The model under review builds one solid part; all positions refer to its coordinate system, in mm. A direction names the side the tool comes from. Give positions to 0.01 mm unless a question says otherwise; leave off trailing zeros. Loops run counter-clockwise (first coordinate to the right, second up) from the corner with the lowest first, then second, coordinate; pieces in that order, holes last. Notation, with made-up numbers: M 67,20.5 L 76,20.5 A31 cw 76,56.5 Z; hole C -13,-10 d8. An arc over 180 degrees is marked long. Return JSON: item names as keys, results as strings. Group by question number.
```python
from build123d import *

# Parameters (mm, degrees)
BOSS_EXTRUDE1_DEPTH                       = 10.668
CSK_FOR_6_FLAT_HEAD_MACHINE_SCREW_2_COUNT = 2
CSK_FOR_6_FLAT_HEAD_MACHINE_SCREW_2_PITCH = 29.9974
SKETCH4_R                                 = 1.238307914
CUT_EXTRUDE1_DEPTH                        = 2540


with BuildPart() as part:
    # Sketch1 → Boss-Extrude1 (new body)
    with BuildSketch(Plane.XY.offset(21.5138)):
        with BuildLine():
            Line((9.7663, 28.448), (-1.8923, 28.448))
            Line((-1.8923, 28.448), (-1.8923, 25.4))
            Line((-1.8923, 25.4), (40.0177, 25.4))
            Line((40.0177, 25.4), (40.0177, 28.448))
            Line((40.0177, 28.448), (28.3591, 28.448))
            ThreePointArc((28.3591, 28.448), (23.537953793, 31.499872647), (24.233689565, 37.163204629))
            ThreePointArc((24.233689565, 37.163204629), (23.84595434, 40.870617487), (20.55495, 42.6212))
            Line((20.55495, 42.6212), (17.57045, 42.6212))
            ThreePointArc((17.57045, 42.6212), (14.27944566, 40.870617487), (13.891710435, 37.163204629))
            ThreePointArc((13.891710435, 37.163204629), (14.587446207, 31.499872647), (9.7663, 28.448))
        make_face()
    extrude(amount=-BOSS_EXTRUDE1_DEPTH)

    # Sketch2 → CSK for #6 Flat Head Machine Screw (100)1 (revolve, cut)
    with BuildSketch(Plane(origin=(34.0614, 28.448, 16.1798), x_dir=(0, 0, 1), z_dir=(1, 0, 0))):
        Polygon((0, 0), (0, 3.048), (2.1082, 3.048), (2.1082, 2.844805148), (4.1275, 0), align=None)
    csk_for_6_flat_head_machine_screw_100 = revolve(axis=Axis((34.0614, 34.798, 16.1798), (0, -1, 0)), mode=Mode.SUBTRACT)

    # CSK for _6 Flat Head Machine Screw _ 2: CSK for #6 Flat Head Machine Screw (100)1 ×2
    with Locations(*[(-i * CSK_FOR_6_FLAT_HEAD_MACHINE_SCREW_2_PITCH, 0, 0) for i in range(1, CSK_FOR_6_FLAT_HEAD_MACHINE_SCREW_2_COUNT)]):
        add(csk_for_6_flat_head_machine_screw_100, mode=Mode.SUBTRACT)

    # Sketch4 → Cut-Extrude1 (cut)
    with BuildSketch(Plane(origin=(0, 0, 0), x_dir=(0, 0, -1), z_dir=(1, 0, 0))):
        with Locations(Location((-16.1798, 38.109028288, 0), (0, 0, 229.800644601))):
            Circle(SKETCH4_R)
    extrude(amount=CUT_EXTRUDE1_DEPTH, mode=Mode.SUBTRACT)


solid = part.part
```
(1) Add section C-C (y = 30.75). Write out the cut boundary in (x, z), and give its area (3 significant figures).
(2) For pin 1 (3 mm diameter, centred on y = 38.11, z = 16.18, fed in from +X); pin 2 (1 mm diameter, centred on y = 35.5, z = 18, fed in from -X); pin 3 (5.5 mm diameter, centred on x = 6.5, z = 17.5, fed in from +Y), all flat-tipped, find the tip position at first contact; note any pin that passes through.
(3) Add section B-B (x = 9). Write out the cut boundary in (y, z).
(4) Add section A-A (y = 27.75). Write out the cut boundary in (x, z), and give its area (3 significant figures).
(5) For probe 1 along Y at (x, z) = (19, 15.25); probe 2 along Y at (x, z) = (10, 14), list the stretches that pass through material, from the lowest coordinate up.
(6) Mouldability with a two-part tool opening along Y and no side actions: class faces 4 (the flat face through (-1.892, 27, 16)), 5 (the cylindrical face through (14.3, 40.9, 16.3)), 6 (the conical face through (31.846, 25.781, 15.889)) as released by +Y, released by -Y, zero draft, split by the parting line, or undercut.
(7) For faces 1 (the flat face through (38.2, 28.448, 17.4)), 2 (the flat face through (1, 28.448, 20)), 3 (the flat face through (19, 30, 21.514)), list the 3-axis set-ups (+Z, -Z, +X, -X, +Y, -Y) from which the entire face can be reached by the end or side of a thin tool; tool diameter is ignored.
Verdict:
{
 "1": {"outline": "M 14.15,10.85 L 23.97,10.85 L 23.97,21.51 L 14.15,21.51 Z", "area": "105 mm²"},
 "2": {"pin 1": "stops at x = 24.52", "pin 2": "stops at x = 14.62", "pin 3": "stops at y = 28.45"},
 "3": {"outline": "M 25.4,10.85 L 28.45,10.85 L 28.45,21.51 L 25.4,21.51 Z"},
 "4": {"outline": "M -1.89,10.85 L 40.02,10.85 L 40.02,21.51 L -1.89,21.51 Z; hole C 4.06,16.18 d7.26; hole C 34.06,16.18 d7.26", "area": "364 mm²"},
 "5": {"probe 1": "y = 25.4 to 37.29, 38.93 to 42.62", "probe 2": "y = 25.4 to 28.45"},
 "6": {"face 4": "zero draft", "face 5": "undercut", "face 6": "released by +Y"},
 "7": {"face 1": "+Z, -Z, +X, +Y", "face 2": "+Z, -Z, -X, +Y", "face 3": "+Z, +X, -X, +Y, -Y"}
}
